from build123d import *

# Parameters (mm, degrees)
SKETCH1_W            = 88.9
SKETCH1_H            = 38.1
BOSS_EXTRUDE1_DEPTH  = 3.175
M4_CLEARANCE_HOLE1_D = 4.5
M8_CLEARANCE_HOLE1_D = 9


with BuildPart() as part:
    # Sketch1 → Boss-Extrude1 (new body)
    with BuildSketch(Plane.XY):
        Rectangle(SKETCH1_W, SKETCH1_H)
    extrude(amount=-BOSS_EXTRUDE1_DEPTH)

    # M4 Clearance Hole1 (through all)
    with Locations(Plane.XY):
        with Locations((0, 0)):
            Hole(M4_CLEARANCE_HOLE1_D / 2)

    # M8 Clearance Hole1 (through all)
    with Locations(Plane.XY):
        with Locations((-25.5, 0), (25.5, 0)):
            Hole(M8_CLEARANCE_HOLE1_D / 2)


solid = part.part
Geometry check sheet. Reference: the model listing, model coordinates, mm. Round coordinates to 2 decimals unless told otherwise and drop trailing zeros. Write each loop counter-clockwise with the first axis right and the second up, starting at its lowest first coordinate (ties: lowest second). Pieces come first, ordered by that corner, then holes. Notation, with made-up numbers: (75, -12) -> (122, -12) arc R33 cw to (122, 24) -> close; hole circle Ø5 at (31, 76.25). An arc over 180 degrees is marked (long way). One line per item, written item: value. Start each with the question number.
(1) Draft check along X on faces 1 (the flat face through (-1, 19.05, -2)), 2 (the cylindrical face through (0.29, 2.23, -1.61)), 3 (the cylindrical face through (-21, 0, -2)), 4 (the flat face through (-44.45, 0, -2)). Enter one of: +X half, -X half, draft (parallel to the pull), parting line (faces both ways), or undercut.
(2) Cross-section at D-D, the plane x = 0. Record the cut outline in (y, z) (3 decimals), and give its area (3 significant figures).
(3) Scan lines: line 1 (Y direction, x = 25.5, z = -1.9); line 2 (Y direction, x = 0, z = -0.65); line 3 (X direction, y = 2.5, z = -0.9). Record each from-to range of solid material in increasing order. Write a range as [from, to].
(4) Go/stop test with a flat-tipped pin: pin 1 Ø11.5 at (x, y) = (-25.5, 0) entering from -Z (3 decimals). Record where the tip stops, or that it passes through.
(5) Cross-section at C-C, the plane z = -0.85. Record the cut outline in (x, y), and give its area (3 significant figures).
(6) Cross-section at B-B, the plane y = 0. Record the cut outline in (x, z) (3 decimals).
(7) Cross-section at A-A, the plane x = -25.5. Record the cut outline in (y, z) (3 decimals).
Answer:
1. face 1: draft
1. face 2: undercut
1. face 3: undercut
1. face 4: -X half
2. outline: (-19.05, -3.175) -> (-2.25, -3.175) -> (-2.25, 0) -> (-19.05, 0) -> close; (2.25, -3.175) -> (19.05, -3.175) -> (19.05, 0) -> (2.25, 0) -> close
2. area: 107 mm²
3. line 1: [-19.05, -4.5], [4.5, 19.05]
3. line 2: [-19.05, -2.25], [2.25, 19.05]
3. line 3: [-44.45, -29.24], [-21.76, 21.76], [29.24, 44.45]
4. pin 1: z = -3.175
5. outline: (-44.45, -19.05) -> (44.45, -19.05) -> (44.45, 19.05) -> (-44.45, 19.05) -> close; hole circle Ø9 at (-25.5, 0); hole circle Ø4.5 at (0, 0); hole circle Ø9 at (25.5, 0)
5. area: 3,240 mm²
6. outline: (-44.45, -3.175) -> (-30, -3.175) -> (-30, 0) -> (-44.45, 0) -> close; (-21, -3.175) -> (-2.25, -3.175) -> (-2.25, 0) -> (-21, 0) -> close; (2.25, -3.175) -> (21, -3.175) -> (21, 0) -> (2.25, 0) -> close; (30, -3.175) -> (44.45, -3.175) -> (44.45, 0) -> (30, 0) -> close
7. outline: (-19.05, -3.175) -> (-4.5, -3.175) -> (-4.5, 0) -> (-19.05, 0) -> close; (4.5, -3.175) -> (19.05, -3.175) -> (19.05, 0) -> (4.5, 0) -> close
